Geometry: see drawing. Coordinates: mm, zero at the bounding-box minimum. A direction names the side the tool comes from. Round coordinates to 2 decimals unless told otherwise and drop trailing zeros. Write each loop counter-clockwise with the first axis right and the second up, starting at its lowest first coordinate (ties: lowest second). Pieces come first, ordered by that corner, then holes.
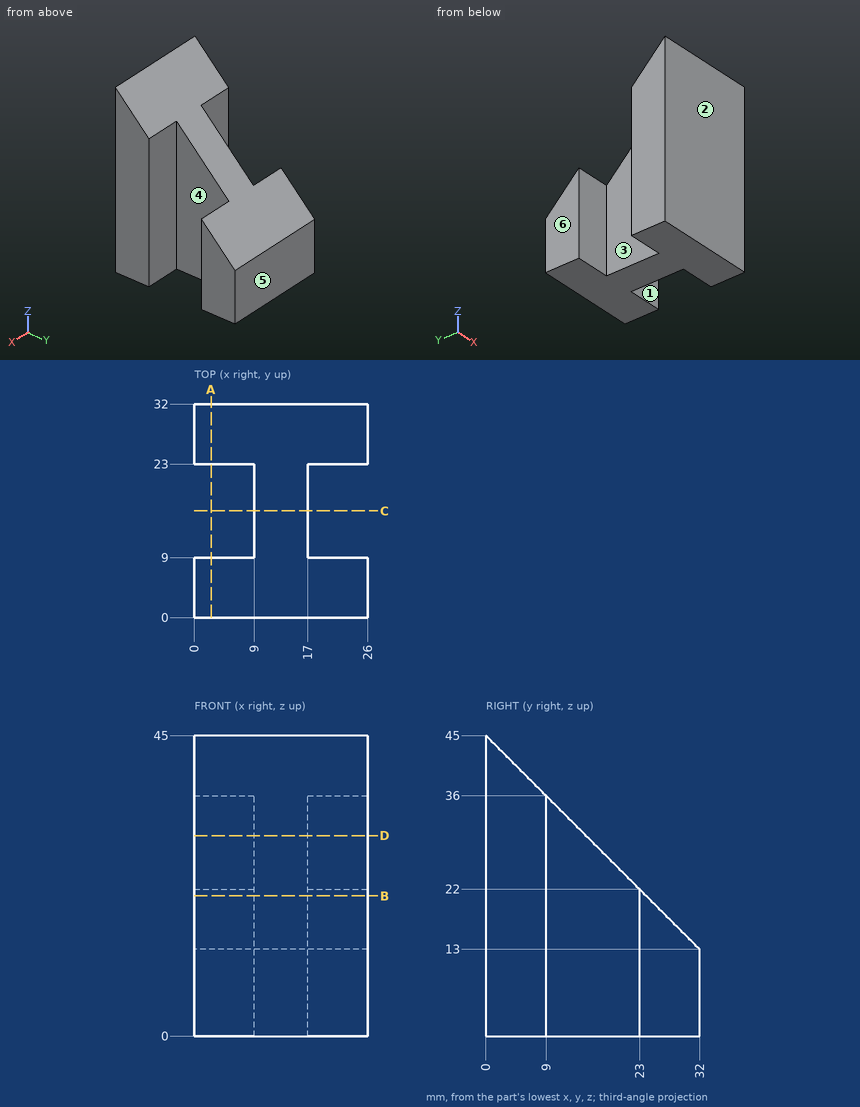
Q1. Set-up query: the marked faces 1, 2 and 3. Return all of +Z, -Z, +X, -X, +Y, -Y with unobstructed straight access to the full face (end or side cutting, diameter ignored); none if empty.
Q2. Section query A-A, the plane x = 2.5. Output: boundary loops of the cut face in (y, z).
Q3. Line query: line 1 (Y direction, x = 8.25, z = 19); line 2 (Y direction, x = 22, z = 4); line 3 (Y direction, x = 17.75, z = 22.5). Output: solid intervals per line, ascending.
Q4. Pin query (flat end, axial travel): P1, Ø4, axis at y = 13, z = 20, coming from the +X side; P2, Ø4, axis at y = 19, z = 25, coming from the -X side. Return the tip coordinate at first contact, or that it passes through.
Q5. Section query B-B, the plane z = 21. Output: boundary loops of the cut face in (x, y).
Q6. Section query D-D, the plane z = 30. Output: boundary loops of the cut face in (x, y), and give its area (3 significant figures).
Q7. Mould query, pull axis Y, two halves, no side actions, for the marked faces 4, 5 and 6. Classes: pulls with the +Y half, pulls with the -Y half, needs draft (parallel to the pull), parting line crosses it, or undercut.
Q8. Section query C-C, the plane y = 16. Output: boundary loops of the cut face in (x, z).
Filled in:
1. face 1: +Z, -Z, +X
1. face 2: +Z, -Z, +X, -X, -Y
1. face 3: +Z, -Z, -X
2. outline: (0, 0) - (9, 0) - (9, 36) - (0, 45) - close; (23, 0) - (32, 0) - (32, 13) - (23, 22) - close
3. line 1: y = 0 to 9, 23 to 26
3. line 2: y = 0 to 9, 23 to 32
3. line 3: y = 0 to 9
4. P1: stops at x = 17
4. P2: stops at x = 9
5. outline: (0, 0) - (26, 0) - (26, 9) - (17, 9) - (17, 23) - (26, 23) - (26, 24) - (0, 24) - (0, 23) - (9, 23) - (9, 9) - (0, 9) - close
6. outline: (0, 0) - (26, 0) - (26, 9) - (17, 9) - (17, 15) - (9, 15) - (9, 9) - (0, 9) - close
6. area: 282 mm2
7. face 4: undercut
7. face 5: pulls with the +Y half
7. face 6: needs draft
8. outline: (9, 0) - (17, 0) - (17, 29) - (9, 29) - close
